Verification items for the finished model (mm, model axes). A direction names the side the tool comes from. Round coordinates to 2 decimals unless told otherwise and drop trailing zeros. Write each loop counter-clockwise with the first axis right and the second up, starting at its lowest first coordinate (ties: lowest second). Pieces come first, ordered by that corner, then holes. Notation, with made-up numbers: M -36.75,0.5 L -13.75,0.5 A31 cw -13.75,26.5 Z; hole C 45.25,56.25 d5. An arc over 180 degrees is marked long. One line per item, written item: value. Start each with the question number.
Item 1: Section check C-C, the plane x = 0. Record the cut outline in (y, z).
Item 2: Section check A-A, the plane y = 0. Record the cut outline in (x, z), then the cut area to 3 significant figures.
Item 3: Section check D-D, the plane z = 25.4. Record the cut outline in (x, y).
Item 4: Thickness scan on probe 1 along Y at (x, z) = (0, 30); probe 2 along Y at (x, z) = (-27, 37.5); probe 3 along X at (y, z) = (-17, 12). Record the ranges inside material, lowest first. Write a range as from..to.
Item 5: Draft check along Y on faces 1 (the face through (148.142, -6, 25)), 2 (the face through (192.971, -56.228, 29.215)), 3 (the face through (239.074, -69, 26)), 4 (the face through (32, -106.441, 25)). Enter one of: +Y half, -Y half, draft (parallel to the pull), parting line (faces both ways), or undercut.
Item 6: Gauge pin test, flat end, axial feed: pin 1 (15 mm diameter, centred on y = -10, z = 37, fed in from +X). Record the tip position at first contact, or that the pin passes through.
Item 7: Section check B-B, the plane z = 43.5. Record the cut outline in (x, y).
Item 8: Tool access check on faces 5 (the face through (-98.615, 89.121, 25.756)), 6 (the face through (192.971, 55.654, 25.958)). Record the directions out of +Z, -Z, +X, -X, +Y, -Y that give a thin tool (end or side, any length) a straight path to the whole face; none if there is none.
from build123d import *

# Parameters (mm, degrees)
F0_W     = 254
F0_H     = 203.2
F0_R     = 63.5
F1_DEPTH = 50.8
F2_R     = 25.4
F3_R     = 12.7
F4_DEPTH = 90.932


with BuildPart() as f1:
    # F0 (on Top) → F1 (new body)
    with BuildSketch(Plane.XY):
        with Locations((21.141905, -4.841334)):
            Rectangle(F0_W, F0_H)
        Circle(F0_R, mode=Mode.SUBTRACT)
    extrude(amount=F1_DEPTH)

    # F2
    f2_edges = [f1.edges().sort_by_distance(p)[0] for p in [
        (-105.858095, 96.758666, 25.4),
        (-105.858095, -106.441334, 25.4),
    ]]
    fillet(f2_edges, radius=F2_R)

    # F3 (on face) → F4 (join)
    with BuildSketch(Plane.YZ.offset(148.141905)):
        with Locations((-68.341334, 25.4)):
            Circle(F3_R)
        with Locations((68.341334, 25.4)):
            Circle(F3_R)
    extrude(amount=F4_DEPTH)


solid = f1.part
Response values:
1. outline: M -106.44,0 L -63.5,0 L -63.5,50.8 L -106.44,50.8 Z; M 63.5,0 L 96.76,0 L 96.76,50.8 L 63.5,50.8 Z
2. outline: M -105.86,0 L -63.5,0 L -63.5,50.8 L -105.86,50.8 Z; M 63.5,0 L 148.14,0 L 148.14,50.8 L 63.5,50.8 Z
2. area: 6,450 mm2
3. outline: M -105.86,-81.04 A25.4 ccw -80.46,-106.44 L 148.14,-106.44 L 148.14,-81.04 L 239.07,-81.04 L 239.07,-55.64 L 148.14,-55.64 L 148.14,55.64 L 239.07,55.64 L 239.07,81.04 L 148.14,81.04 L 148.14,96.76 L -80.46,96.76 A25.4 ccw -105.86,71.36 Z; hole C 0,0 d127
4. probe 1: y = -106.44..-63.5, 63.5..96.76
4. probe 2: y = -106.44..-57.47, 57.47..96.76
4. probe 3: x = -105.86..-61.18, 61.18..148.14
5. face 1: undercut
5. face 2: undercut
5. face 3: draft
5. face 4: -Y half
6. pin 1: stops at x = 148.14
7. outline: M -105.86,-81.04 A25.4 ccw -80.46,-106.44 L 148.14,-106.44 L 148.14,96.76 L -80.46,96.76 A25.4 ccw -105.86,71.36 Z; hole C 0,0 d127
8. face 5: +Z, -Z, -X, +Y
8. face 6: +X
